The listing builds one solid part. Answer for the finished solid, in the listing's coordinates (mm). Face numbers are marked on the shaded views. Give positions to 0.01 mm unless a question says otherwise; leave off trailing zeros. Loops run counter-clockwise (first coordinate to the right, second up) from the corner with the lowest first, then second, coordinate; pieces in that order, holes last. Notation, with made-up numbers: (78, -26.75) - (132, -26.75) arc R24 ccw to (132, 11.25) - close; hole circle Ø10 at (-17, 32.25). An arc over 180 degrees is marked (long way). Write item = value, one per line. Start each with the question number.
1) The part is cut by section C-C on y = 14.2. Write down the section's boundary in (x, z), plus the area to 3 significant figures.
2) The part is cut by section B-B on z = 2.75. Write down the section's boundary in (x, y), plus the area to 3 significant figures.
3) Consider probe 1 along X at (y, z) = (17, -0.25); probe 2 along Z at (x, y) = (1.45, 6.6); probe 3 along Z at (x, y) = (0.55, -0.75). Determine where each line is inside the solid, lowest interval first.
4) The part is cut by section A-A on y = 4.7. Write down the section's boundary in (x, z), plus the area to 3 significant figures.
5) The mould has two halves that part along Y. Classify the marked faces 1, 2 and 3: +Y half, -Y half, draft (parallel to the pull), parting line (faces both ways), or undercut.
6) Flat-ended cylindrical pins translate along their axes: P1, Ø2, axis at x = 1.5, y = 3, coming from the -Z side; P2, Ø3.5, axis at y = 0, z = 0, coming from the +X side; P3, Ø1.5, axis at x = 1, y = 7.5, coming from the +Z side. Find the tip coordinate at first contact, or state that the pin passes through.
from build123d import *

# Parameters (mm, degrees)
SKETCH079_R        = 3.4
PAD047_DEPTH       = 4.8
PAD048_DEPTH       = 2.15
POCKET033_DEPTH    = 3
POLARPATTERN_COUNT = 20
SKETCH082_R        = 2.4
POCKET034_DEPTH    = 1
SKETCH083_R        = 1.3
POCKET035_DEPTH    = 5
SKETCH084_R        = 0.5
POCKET036_DEPTH    = 5


with BuildPart() as part:
    # Sketch079 → Pad047 (new body)
    with BuildSketch(Plane.YZ):
        Circle(SKETCH079_R)
    extrude(amount=PAD047_DEPTH)

    # Sketch080 → Pad048 (join)
    with BuildSketch(Plane.YZ.offset(0.5)):
        with BuildLine():
            ThreePointArc((16.175, -1.9923290391), (18, 0), (16.175, 1.9923290391))
            Line((0.2975, 3.3869593665), (16.175, 1.9923290391))
            ThreePointArc((0.2975, 3.3869593665), (-3.4, 0), (0.2975, -3.3869593665))
            Line((0.2975, -3.3869593665), (16.175, -1.9923290391))
        make_face()
    extrude(amount=PAD048_DEPTH)

    # Sketch081 (on Face10 of Pad048) → Pocket033 (cut)
    with BuildSketch(Plane.YZ.offset(4.8)):
        with BuildLine():
            Line((2.4, 0), (1.9234666187, -0.1513801059))
            Line((1.9234666187, -0.1513801059), (2.3704520174, -0.3754427161))
            Line((0, 0), (2.3704520174, -0.3754427161))
            Line((2.3704520174, 0.3754427161), (0, 0))
            ThreePointArc((2.4, 0), (2.392601601, 0.1883018297), (2.3704520174, 0.3754427161))
        make_face()
    pocket033 = extrude(amount=-POCKET033_DEPTH, mode=Mode.SUBTRACT)

    # PolarPattern: Pocket033 ×20 about axis
    polarpattern_axis = Axis((4.8, 0, 0), (1, 0, 0))
    for i in range(1, POLARPATTERN_COUNT):
        add(pocket033.rotate(polarpattern_axis, i * 360 / POLARPATTERN_COUNT), mode=Mode.SUBTRACT)

    # Sketch082 (on Face2 of PolarPattern) → Pocket034 (cut)
    with BuildSketch(Plane(origin=(0, 0, 0), x_dir=(0, 1, 0), z_dir=(-1, 0, 0))):
        Circle(SKETCH082_R)
    extrude(amount=-POCKET034_DEPTH, mode=Mode.SUBTRACT)

    # Sketch083 (on Face10 of Pocket034) → Pocket035 (cut)
    with BuildSketch(Plane(origin=(1, 0, 0), x_dir=(0, 1, 0), z_dir=(-1, 0, 0))):
        Circle(SKETCH083_R)
    extrude(amount=-POCKET035_DEPTH, mode=Mode.SUBTRACT)

    # Sketch084 (on Face3 of Pocket035) → Pocket036 (cut)
    with BuildSketch(Plane(origin=(0.5, 0, 0), x_dir=(0, 1, 0), z_dir=(-1, 0, 0))):
        with Locations((4.7, 0)):
            Circle(SKETCH084_R)
        with Locations((6.6, 0)):
            Circle(SKETCH084_R)
        with Locations((8.5, 0)):
            Circle(SKETCH084_R)
        with Locations((10.4, 0)):
            Circle(SKETCH084_R)
        with Locations((12.3, 0)):
            Circle(SKETCH084_R)
        with Locations((14.2, 0)):
            Circle(SKETCH084_R)
        with Locations((16.1, 0)):
            Circle(SKETCH084_R)
    extrude(amount=-POCKET036_DEPTH, mode=Mode.SUBTRACT)


solid = part.part
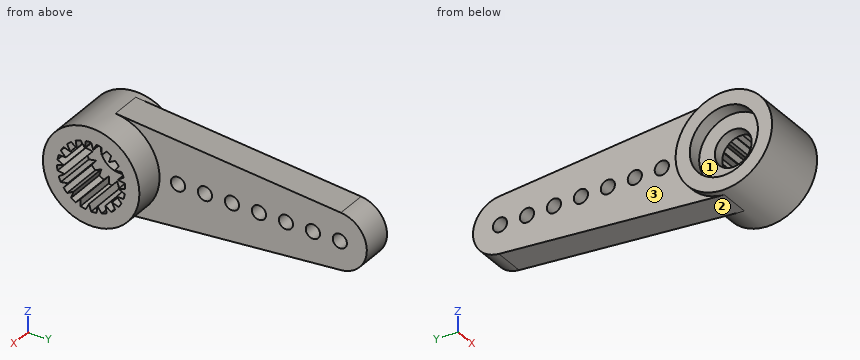
Answer below:
q1.outline = (0.5, -2.17) - (2.65, -2.17) - (2.65, -0.5) - (0.5, -0.5) - close; (0.5, 0.5) - (2.65, 0.5) - (2.65, 2.17) - (0.5, 2.17) - close
q1.area = 7.16 mm2
q2.outline = (0, -2) - (4.8, -2) - (4.8, 2) - (2.65, 2) - (2.65, 7.55) - (0.5, 7.55) - (0.5, 2) - (0, 2) - close
q2.area = 31.1 mm2
q3.probe_1 = 0.5 to 2.65
q3.probe_2 = -2.83 to -0.5, 0.5 to 2.83
q3.probe_3 = -3.32 to -2.28, 2.28 to 3.32
q4.outline = (0.5, -3) - (2.65, -3) - (2.65, -0.5) - (0.5, -0.5) - close; (0.5, 0.5) - (2.65, 0.5) - (2.65, 3) - (0.5, 3) - close
q4.area = 10.8 mm2
q5.face_1 = undercut
q5.face_2 = +Y half
q5.face_3 = draft
q6.P1 = -3.24
q6.P2 = 1.8
q6.P3 = 2.82
